Read the model definition and answer for the solid it produces. Units are mm, in the model's axes. Round coordinates to 2 decimals unless told otherwise and drop trailing zeros. Order: outer loops, then holes, each group sorted by start corner. A loop starts at its lowest first (then second) coordinate and runs counter-clockwise, first axis right, second up. Notation, with made-up numbers: M 23.25,-22 L 38.25,-22 A19 ccw 38.25,-14 Z; hole C -36,-32 d7. An arc over 180 degrees is marked long. Answer as CSV lines item,"result".
```python
from build123d import *

# Parameters (mm, degrees)
BOX_W                  = 70
BOX_H                  = 200
BOX_DEPTH              = 11.6
POCKET_DEPTH           = 200.001
LINEARPATTERN_COUNT    = 5
LINEARPATTERN_PITCH    = 14.5
SKETCH_W               = 82.408782
SKETCH_H               = 38.885188
SKETCH_W_2             = 6
SKETCH_H_2             = 21.094656
POCKET001_DEPTH        = 200.001
SKETCH003_R            = 1
POCKET002_DEPTH        = 5.201
LINEARPATTERN001_COUNT = 3
LINEARPATTERN001_PITCH = 15


with BuildPart() as part:
    # Box → Box (new body)
    with BuildSketch(Plane(origin=(-7.5, 0, 0), x_dir=(1, 0, 0), z_dir=(0, 0, 1))):
        with Locations((35, 100)):
            Rectangle(BOX_W, BOX_H)
    extrude(amount=BOX_DEPTH)

    # Sketch002 → Pocket (cut, through all)
    with BuildSketch(Plane(origin=(-7.5, 0, 0), x_dir=(1, 0, 0), z_dir=(0, -1, 0))):
        Polygon((14.1, 10), (11.2, 10), (11.2, 3), (2.7, 3), (2.7, 10), (1.9, 10), (1.9, 10.4), (2.25, 11.6), (13.75, 11.6), (14.1, 10.4), align=None)
    pocket = extrude(amount=-POCKET_DEPTH, mode=Mode.SUBTRACT)

    # LinearPattern: Pocket ×5
    with Locations(*[(i * LINEARPATTERN_PITCH, 0, 0) for i in range(1, LINEARPATTERN_COUNT)]):
        add(pocket, mode=Mode.SUBTRACT)

    # Sketch → Pocket001 (cut, through all)
    with BuildSketch(Plane(origin=(-7.5, 0, 0), x_dir=(1, 0, 0), z_dir=(0, -1, 0))):
        with Locations((35.413628, 6.289411)):
            Rectangle(SKETCH_W, SKETCH_H)
        with Locations((14.2, 4.644143)):
            Rectangle(SKETCH_W_2, SKETCH_H_2, mode=Mode.SUBTRACT)
    extrude(amount=-POCKET001_DEPTH, mode=Mode.SUBTRACT)

    # Sketch003 → Pocket002 (cut, through all)
    with BuildSketch(Plane.YZ.offset(8.9)):
        with Locations((21.45, -100)):
            Circle(SKETCH003_R)
        with Locations((21.45, -10)):
            Circle(SKETCH003_R)
        with Locations((21.45, -190)):
            Circle(SKETCH003_R)
    pocket002 = extrude(amount=-POCKET002_DEPTH, mode=Mode.SUBTRACT)

    # LinearPattern001: Pocket002 ×3
    with Locations(*[(0, i * LINEARPATTERN001_PITCH, 0) for i in range(1, LINEARPATTERN001_COUNT)]):
        add(pocket002, mode=Mode.SUBTRACT)


solid = part.part
```
Item 1: A cutting plane is placed at A-A, the plane y = 58.5. Determine the outline of the cut face in (x, z).
Ans:
outline,"M 3.7,0 L 9.7,0 L 9.7,10 L 8.9,10 L 8.9,10.4 L 9.25,11.6 L 6.25,11.6 L 6.6,10.4 L 6.6,10 L 3.7,10 Z"
Item 2: Find the intervals of material crossed by probe 1 along Z at (x, y) = (4.35, 23); probe 2 along X at (y, z) = (188.5, 10.25), in increasing order. Write a range as [from, to].
Ans:
probe 1,"[0, 10]"
probe 2,"[6.6, 8.9]"
Item 3: A cutting plane is placed at B-B, the plane x = 4.6. Determine the outline of the cut face in (y, z), and give its area (3 significant figures).
Ans:
outline,"M 0,0 L 200,0 L 200,10 L 0,10 Z"
area,"2,000 mm2"
